```python
from build123d import *

# Parameters (mm, degrees)
F2_W      = 1.2519505165
F2_H      = 13
F3_DEPTH  = 15
F4_R      = 5
F5_R      = 1
F6_R      = 3.05
F7_DEPTH  = 13
F8_R      = 0.5
F10_R     = 1.2
F11_DEPTH = 12.5


with BuildPart() as f1:
    # F0 (on Front) → F1 (revolve)
    with BuildSketch(Plane.XZ):
        Polygon((-5, 0), (0, 0), (0, 15), (-6.5, 15), (-6.5, 0), align=None)
    revolve(axis=Axis((0, 0, -3.6677676575), (0, 0, -1)))

    # F2 (on Top) → F3 (join)
    with BuildSketch(Plane.XY):
        with BuildLine():
            Line((0, -6.5), (0, 6.5))
            ThreePointArc((0, 6.5), (-6.5, 0), (0, -6.5))
        make_face()
        with Locations((0.6259752583, 0)):
            Rectangle(F2_W, F2_H)
        Polygon((15, 1), (1.2519505165, 6.5), (1.2519505165, -6.5), (15, -1), align=None)
    extrude(amount=F3_DEPTH)

    # F4
    f4_edges = [f1.edges().sort_by_distance(p)[0] for p in [
        (1.251951, 6.5, 7.5),
        (1.251951, -6.5, 7.5),
    ]]
    fillet(f4_edges, radius=F4_R)

    # F5
    f5_edges = [f1.edges().sort_by_distance(p)[0] for p in [
        (15, 1, 7.5),
        (15, -1, 7.5),
    ]]
    fillet(f5_edges, radius=F5_R)

    # F6 (on face) → F7 (cut)
    with BuildSketch(Plane(origin=(0, 0, 0), x_dir=(1, 0, 0), z_dir=(0, 0, -1))):
        Circle(F6_R)
    extrude(amount=-F7_DEPTH, mode=Mode.SUBTRACT)

    # F8
    f8_edges = [f1.edges().sort_by_distance(p)[0] for p in [
        (8.258764, -3.696877, 15),
        (14.828081, -0.883611, 15),
        (1.234569, -6.409759, 15),
        (15, 0, 15),
        (0.144456, -6.5, 15),
        (14.828081, 0.883611, 15),
        (-6.5, 0, 15),
        (8.258764, 3.696877, 15),
        (0.144456, 6.5, 15),
        (1.234569, 6.409759, 15),
    ]]
    fillet(f8_edges, radius=F8_R)

    # F10 (on line) → F11 (cut, symmetric)
    with BuildSketch(Plane(origin=(0, 0, 0), x_dir=(-0.7071067812, -0.7071067812, 0), z_dir=(-0.7071067812, 0.7071067812, 0))):
        with Locations((0, 9)):
            Circle(F10_R)
    extrude(amount=F11_DEPTH, both=True, mode=Mode.SUBTRACT)


solid = f1.part
```
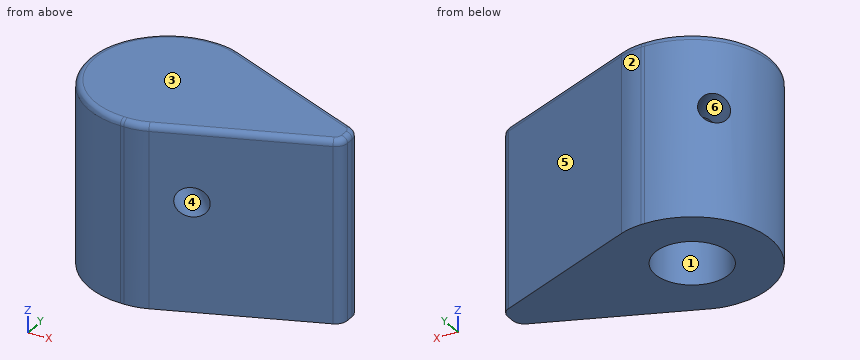
Build history of the part. All positions in model axes, mm. Face numbers are marked on the shaded views. A direction names the side the tool comes from. Round coordinates to 2 decimals unless told otherwise and drop trailing zeros. Write each loop counter-clockwise with the first axis right and the second up, starting at its lowest first coordinate (ties: lowest second). Pieces come first, ordered by that corner, then holes.
1) Band-saw the part on A-A, the plane z = 7.5. List the corners of the cut face in (x, y), and give its area (3 significant figures).
2) Band-saw the part on B-B, the plane y = 0. List the corners of the cut face in (x, z).
3) Drill centre lines: probe 1 along X at (y, z) = (0, 9.5); probe 2 along Y at (x, z) = (-2.75, 8); probe 3 along Y at (x, z) = (-0.75, 7.5). Where is each one in solid material? Low to high.
4) 3-axis set-ups, long thin cutter, end or side, ignore diameter. For the marked faces 1 and 2: which of +Z, -Z, +X, -X, +Y, -Y reach the whole face in a straight line?
5) Band-saw the part on C-C, the plane z = 9.25. List the corners of the cut face in (x, y).
6) Pin check, flat tips, straight feed: pin 1 (2 mm diameter, centred on y = -2.5, z = 13, fed in from +X); pin 2 (1.5 mm diameter, centred on y = 4.5, z = 2, fed in from +X); pin 3 (1.5 mm diameter, centred on y = 4, z = 3, fed in from +X). Stop position of each tip, or through.
7) Mould opens along X. For the marked faces 3, 4, 5 and 6 say: +X half, -X half, draft (parallel to the pull), parting line (faces both ways), or undercut.
Ans:
1. outline: (0, -6.5) - (0.29, -6.5) arc R5 ccw to (2.15, -6.14) - (14.37, -1.25) arc R1 ccw to (15, -0.32) - (15, 0.32) arc R1 ccw to (14.37, 1.25) - (2.15, 6.14) arc R5 ccw to (0.29, 6.5) - (0, 6.5) arc R6.5 ccw to start; hole circle Ø6.1 at (0, 0)
1. area: 156 mm2
2. outline: (-6.5, 0) - (-3.05, 0) - (-3.05, 13) - (3.05, 13) - (3.05, 0) - (15, 0) - (15, 14.5) arc R0.5 ccw to (14.5, 15) - (-6, 15) arc R0.5 ccw to (-6.5, 14.5) - close
3. probe 1: x = -6.5 to -3.05, 3.05 to 15
3. probe 2: y = -5.89 to -1.32, 1.32 to 1.81, 3.69 to 5.89
3. probe 3: y = -6.46 to -2.96, 2.96 to 6.46
4. face 1: -Z
4. face 2: +Z, -Z, +X, +Y
5. outline: (-5.35, 3.69) arc R6.5 ccw to (0, -6.5) - (0.29, -6.5) arc R5 ccw to (2.15, -6.14) - (3.81, -5.47) - (1.16, -2.82) arc R3.05 cw to (-2.82, 1.16) - close; (-3.69, 5.35) - (-1.16, 2.82) arc R3.05 cw to (2.82, -1.16) - (6.19, -4.53) - (14.37, -1.25) arc R1 ccw to (15, -0.32) - (15, 0.32) arc R1 ccw to (14.37, 1.25) - (2.15, 6.14) arc R5 ccw to (0.29, 6.5) - (0, 6.5) arc R6.5 ccw to start
6. pin 1: stops at x = 13.75
6. pin 2: stops at x = 8.13
6. pin 3: stops at x = 9.38
7. face 3: draft
7. face 4: undercut
7. face 5: +X half
7. face 6: undercut
